Read the model definition and answer for the solid it produces. Units are mm, in the model's axes. A direction names the side the tool comes from. Coordinates: 2 decimals unless noted, no trailing zeros. Loops run counter-clockwise (first coordinate to the right, second up) from the corner with the lowest first, then second, coordinate; pieces in that order, holes last.
from build123d import *

# Parameters (mm, degrees)
SKETCH_1_R      = 11.025
SKETCH_1_R_2    = 1.5
SKETCH_1_R_3    = 2
SKETCH_1_R_4    = 4
SKETCH_1_W      = 6.2
SKETCH_1_H      = 4.6
EXTRUDE_1_DEPTH = 3


with BuildPart() as part:
    # 草图1 → 凸台-拉伸1 (new body)
    with BuildSketch(Plane(origin=(0, 0, 0), x_dir=(1, 0, 0), z_dir=(0, 1, 0))):
        with BuildLine():
            Line((-4.330127019, 48), (-43.734282891, -20.25))
            ThreePointArc((-43.734282891, -20.25), (-43.734282891, -25.25), (-39.404155872, -27.75))
            Line((-39.404155872, -27.75), (39.404155872, -27.75))
            ThreePointArc((39.404155872, -27.75), (43.734282891, -25.25), (43.734282891, -20.25))
            Line((43.734282891, -20.25), (4.330127019, 48))
            ThreePointArc((4.330127019, 48), (0, 50.5), (-4.330127019, 48))
        make_face()
        with Locations(Location((0, 0, 0), (0, 0, 270))):
            Circle(SKETCH_1_R, mode=Mode.SUBTRACT)
        with Locations(Location((0, 45.5, 0), (0, 0, 270))):
            Circle(SKETCH_1_R_2, mode=Mode.SUBTRACT)
        with Locations(Location((39.404155872, -22.75, 0), (0, 0, 270))):
            Circle(SKETCH_1_R_2, mode=Mode.SUBTRACT)
        with Locations(Location((-39.404155872, -22.75, 0), (0, 0, 270))):
            Circle(SKETCH_1_R_2, mode=Mode.SUBTRACT)
        with Locations(Location((0, 29, 0), (0, 0, 270))):
            Circle(SKETCH_1_R_3, mode=Mode.SUBTRACT)
        with Locations(Location((25.11473671, -14.5, 0), (0, 0, 270))):
            Circle(SKETCH_1_R_3, mode=Mode.SUBTRACT)
        with Locations(Location((-25.11473671, -14.5, 0), (0, 0, 270))):
            Circle(SKETCH_1_R_3, mode=Mode.SUBTRACT)
        with Locations(Location((0, 19.25, 0), (0, 0, 270))):
            Circle(SKETCH_1_R_4, mode=Mode.SUBTRACT)
        Polygon((-12.479611541, 10.784678752), (-16.463328399, 13.084678752), (-19.563328399, 7.715321248), (-15.579611541, 5.415321248), align=None, mode=Mode.SUBTRACT)
        with Locations((0, -18.5)):
            Rectangle(SKETCH_1_W, SKETCH_1_H, mode=Mode.SUBTRACT)
        Polygon((15.579611541, 5.415321248), (19.563328399, 7.715321248), (16.463328399, 13.084678752), (12.479611541, 10.784678752), align=None, mode=Mode.SUBTRACT)
    extrude(amount=EXTRUDE_1_DEPTH)


solid = part.part
Q1. A cutting plane is placed at A-A (z = 22.75). Give the vertices of the cut face in (x, y).
Findings below:
outline: (-44.4, 0) - (-40.9, 0) - (-40.9, 3) - (-44.4, 3) - close; (-37.9, 0) - (37.9, 0) - (37.9, 3) - (-37.9, 3) - close; (40.9, 0) - (44.4, 0) - (44.4, 3) - (40.9, 3) - close
Q2. Determine the mould class of faces 3 (the face through (24.308, 1.479, -13.397)), 4 (the face through (3.1, 1, 19)), 5 (the face through (-10, 0, 5)) for opening direction X: +X half, -X half, draft (parallel to the pull), parting line (faces both ways), or undercut.
Findings below:
face 3: +X half
face 4: undercut
face 5: draft
Q3. Straight lines are drawn through the part: probe 1 along Z at (x, y) = (9, 0.3); probe 2 along Z at (x, y) = (-3, 1.4); probe 3 along X at (y, z) = (1.5, -46.5). For each, find the intervals that lie inside material, in ascending order.
Findings below:
probe 1: z = -39.91 to -6.37, 6.37 to 27.75
probe 2: z = -49.5 to -21.9, -16.6 to -10.61, 10.61 to 16.2, 20.8 to 27.75
probe 3: x = -5.2 to -1.12, 1.12 to 5.2
Q4. A cutting plane is placed at C-C (z = -29). Give the vertices of the cut face in (x, y), then the cut area to 3 significant figures.
Findings below:
outline: (-15.3, 0) - (-2, 0) - (-2, 3) - (-15.3, 3) - close; (2, 0) - (15.3, 0) - (15.3, 3) - (2, 3) - close
area: 79.8 mm2
Q5. Flat-ended cylindrical pins translate along their axes: pin 1 Ø3 at (x, z) = (-25.11, 14.5) entering from +Y; pin 2 Ø1 at (x, y) = (6.5, 1) entering from -Z; pin 3 Ø1.5 at (y, z) = (1, -13) entering from +X. Find the tip coordinate at first contact, or state that the pin passes through.
Findings below:
pin 1: passes through
pin 2: stops at z = -45.11
pin 3: stops at x = 24.97
Q6. A cutting plane is placed at B-B (x = 0). Give the vertices of the cut face in (y, z) (3 decimals), then the cut area to 3 significant figures.
Findings below:
outline: (0, -50.5) - (3, -50.5) - (3, -47) - (0, -47) - close; (0, -44) - (3, -44) - (3, -31) - (0, -31) - close; (0, -27) - (3, -27) - (3, -23.25) - (0, -23.25) - close; (0, -15.25) - (3, -15.25) - (3, -11.025) - (0, -11.025) - close; (0, 11.025) - (3, 11.025) - (3, 16.2) - (0, 16.2) - close; (0, 20.8) - (3, 20.8) - (3, 27.75) - (0, 27.75) - close
area: 110 mm2
Q7. Which of the six approach directions +Z, -Z, +X, -X, +Y, -Y give full straight-line access (tool end or side, diameter ignored) to faces 1 (the face through (18.035, 1.479, -10.362)), 2 (the face through (-23.76, 1.48, -14.35))?
Findings below:
face 1: +Y, -Y
face 2: -Z, -X, +Y, -Y
Q8. A cutting plane is placed at D-D (y = 1.8). Count the separate pieces of the cut face and the enclosed holes in it, then the cut area to 3 significant figures.
Findings below:
separate pieces: 1
enclosed holes: 11
area: 3,370 mm2
